from build123d import *

# Parameters (mm, degrees)
SKETCH1_R      = 9.5
EXTRUDE1_DEPTH = 5


with BuildPart() as part:
    # Sketch1 → Extrude1 (new body)
    with BuildSketch(Plane.XY):
        with BuildLine():
            Line((0, 14), (155, 14))
            ThreePointArc((155, 14), (160.643434486, 13.092444155), (165.717787645, 10.461294133))
            ThreePointArc((165.717787645, 10.461294133), (166.119633231, 9.731618991), (165.829461779, 8.950782122))
            Line((165.829461779, 8.950782122), (163.140222938, 6.261543282))
            ThreePointArc((163.140222938, 6.261543282), (162.527882268, 5.973150498), (161.872126258, 6.140827417))
            ThreePointArc((161.872126258, 6.140827417), (146.33794193, -12.66205807), (165.140827417, 2.872126258))
            ThreePointArc((165.140827417, 2.872126258), (164.973150498, 3.527882268), (165.261543282, 4.140222938))
            Line((165.261543282, 4.140222938), (167.950782122, 6.829461779))
            ThreePointArc((167.950782122, 6.829461779), (168.731618991, 7.119633231), (169.461294133, 6.717787645))
            ThreePointArc((169.461294133, 6.717787645), (172.092444155, 1.643434486), (173, -4))
            Line((173, -4), (173, -34.5))
            ThreePointArc((173, -34.5), (172.682195303, -36.830428123), (171.751990775, -38.990662972))
            ThreePointArc((171.751990775, -38.990662972), (170.973301155, -39.471650118), (170.129341386, -39.117477748))
            Line((170.129341386, -39.117477748), (168.594776555, -37.288654597))
            ThreePointArc((168.594776555, -37.288654597), (168.37185122, -36.79398444), (168.440072921, -36.255709354))
            ThreePointArc((168.440072921, -36.255709354), (161.404162333, -31.052800006), (165.306254745, -38.88529503))
            ThreePointArc((165.306254745, -38.88529503), (165.848198797, -38.911580258), (166.296643225, -39.217017426))
            Line((166.296643225, -39.217017426), (167.831208056, -41.045840577))
            ThreePointArc((167.831208056, -41.045840577), (168.033447677, -41.938480088), (167.424549772, -42.621817122))
            ThreePointArc((167.424549772, -42.621817122), (165.097799098, -43.166346819), (162.710657326, -43.057555971))
            Line((162.710657326, -43.057555971), (105.10076609, -32.38019375))
            ThreePointArc((105.10076609, -32.38019375), (104.458875427, -31.96334508), (104.299746708, -31.214703317))
            Line((104.299746708, -31.214703317), (104.878820837, -28.090298909))
            ThreePointArc((104.878820837, -28.090298909), (105.118722541, -27.603635328), (105.577463168, -27.31389181))
            ThreePointArc((105.577463168, -27.31389181), (105.116766441, -18.575352916), (101.555056728, -26.568382843))
            ThreePointArc((101.555056728, -26.568382843), (101.879493209, -27.003279657), (101.929056114, -27.543592333))
            Line((101.929056114, -27.543592333), (101.349981985, -30.667996741))
            ThreePointArc((101.349981985, -30.667996741), (100.933133315, -31.309887404), (100.184491552, -31.469016123))
            Line((100.184491552, -31.469016123), (8.640568057, -14.502352773))
            ThreePointArc((8.640568057, -14.502352773), (5.918550852, -14.125852173), (3.173502293, -14))
            Line((3.173502293, -14), (0, -14))
            ThreePointArc((0, -14), (-8.89684473, -10.809539946), (-13.738685501, -2.692307692))
            ThreePointArc((-13.738685501, -2.692307692), (-13.529460818, -1.864511091), (-12.757350822, -1.5))
            Line((-12.757350822, -1.5), (-10.198039027, -1.5))
            ThreePointArc((-10.198039027, -1.5), (-9.580825627, -1.713204208), (-9.226797215, -2.261904762))
            ThreePointArc((-9.226797215, -2.261904762), (9.5, 0), (-9.226797215, 2.261904762))
            ThreePointArc((-9.226797215, 2.261904762), (-9.580825627, 1.713204208), (-10.198039027, 1.5))
            Line((-10.198039027, 1.5), (-12.757350822, 1.5))
            ThreePointArc((-12.757350822, 1.5), (-13.529460818, 1.864511091), (-13.738685501, 2.692307692))
            ThreePointArc((-13.738685501, 2.692307692), (-8.89684473, 10.809539946), (0, 14))
        make_face()
        with Locations((30, 0)):
            Circle(SKETCH1_R, mode=Mode.SUBTRACT)
        with Locations((60, 0)):
            Circle(SKETCH1_R, mode=Mode.SUBTRACT)
        with Locations((90, 0)):
            Circle(SKETCH1_R, mode=Mode.SUBTRACT)
        with Locations((120, 0)):
            Circle(SKETCH1_R, mode=Mode.SUBTRACT)
    extrude(amount=EXTRUDE1_DEPTH)


solid = part.part
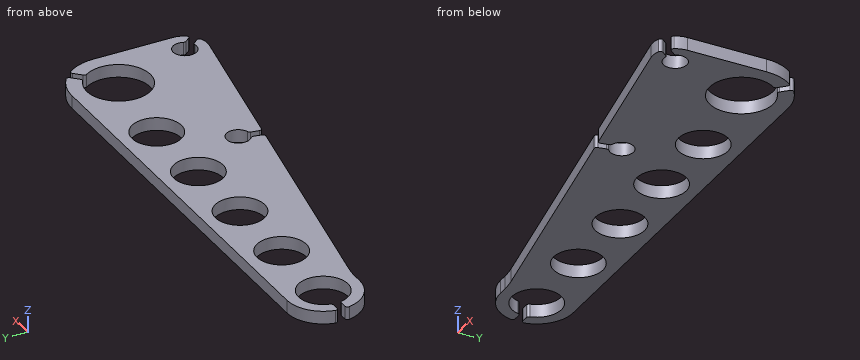
CAD build for the part. Positions are in the model's coordinates, mm. Round coordinates to 2 decimals unless told otherwise and drop trailing zeros. Order: outer loops, then holes, each group sorted by start corner. A loop starts at its lowest first (then second) coordinate and runs counter-clockwise, first axis right, second up. Notation, with made-up numbers: (14, 89.25) -> (72, 89.25) arc R21 cw to (72, 119.25) -> close; hole circle Ø1 at (82, -1.75). An arc over 180 degrees is marked (long way). Write each question's results on one line, items separated by ' | '.
1. Cut at C-C (z = 2.15). Count the separate pieces of the cut face and the enclosed holes in it, plus the area to 3 significant figures.
Findings below:
separate pieces: 1 | enclosed holes: 4 | area: 5,570 mm²
2. Wall check: line 1 along Y through (x, z) = (161.5, 4.55); line 2 along Y through (x, z) = (81.5, 1.75); line 3 along X through (y, z) = (-0.5, 2.4). Give the ranges that are in metal, low to high. Write a range as [from, to].
Findings below:
line 1: y = [-42.83, -38.03], [-30.97, -14.38], [6.38, 12.79] | line 2: y = [-28.01, -4.24], [4.24, 14] | line 3: x = [9.49, 20.51], [39.49, 50.51], [69.49, 80.51], [99.49, 110.51], [129.49, 143.26], [166.74, 172.66]
3. Flat gauge pins, fed straight in: P1, Ø3, axis at x = -11, z = 2, coming from the +Y side; P2, Ø3, axis at x = -12, z = 3, coming from the -Y side; P3, Ø3, axis at x = 73, z = 1.5, coming from the -Y side; P4, Ø3, axis at x = 93, y = -32.5, coming from the +Z side. Where does each tip first touch, or does it go through?
Findings below:
P1: stops at y = 10.28 | P2: stops at y = -9.26 | P3: stops at y = -26.71 | P4: passes through
4. Cut at B-B (x = 30). Give the cut face in (y, z), plus the area to 3 significant figures.
Findings below:
outline: (-18.46, 0) -> (-9.5, 0) -> (-9.5, 5) -> (-18.46, 5) -> close; (9.5, 0) -> (14, 0) -> (14, 5) -> (9.5, 5) -> close | area: 67.3 mm²
5. Cut at A-A (y = -23). Give the cut face in (x, z).
Findings below:
outline: (54.49, 0) -> (99.8, 0) -> (99.8, 5) -> (54.49, 5) -> close; (108.8, 0) -> (173, 0) -> (173, 5) -> (108.8, 5) -> close
6. Cut at D-D (x = 74). Give the cut face in (y, z).
Findings below:
outline: (-26.62, 0) -> (14, 0) -> (14, 5) -> (-26.62, 5) -> close
